The figure shows three views and two pictorial views of one solid part (mm, origin at its lowest corner). Answer the questions. Coordinates: 2 decimals unless noted, no trailing zeros. Loops run counter-clockwise (first coordinate to the right, second up) from the corner with the lowest first, then second, coordinate; pieces in that order, holes last. Notation, with made-up numbers: (23.5, -30) -> (38.5, -30) arc R12 ccw to (38.5, -26) -> close; hole circle Ø3 at (22.25, -37). An arc over 180 degrees is marked (long way). Answer as a JSON object with one key per item and string values. Group by question number.
1) Consider probe 1 along Z at (x, y) = (3, 2.3); probe 2 along X at (y, z) = (2, 32); probe 3 along Z at (x, y) = (2.45, 1.35). Determine where each line is inside the solid, lowest interval first. Write a range as [from, to].
2) Determine the mould class of the marked faces 1, 2, 3 and 4 for opening direction X: released by +X, released by -X, zero draft, split by the parting line, or undercut.
3) A flat-ended cylindrical pin translates along its axis: P1, Ø1, axis at x = 1.5, y = 2, coming from the -Z side. Find the tip coordinate at first contact, or state that the pin passes through.
4) Section A-A, the plane x = 3.8 is taken. Give the vertices of the cut face in (y, z).
5) Section B-B, the plane y = 0.45 is taken. Give the vertices of the cut face in (x, z), plus the area to 3 significant figures.
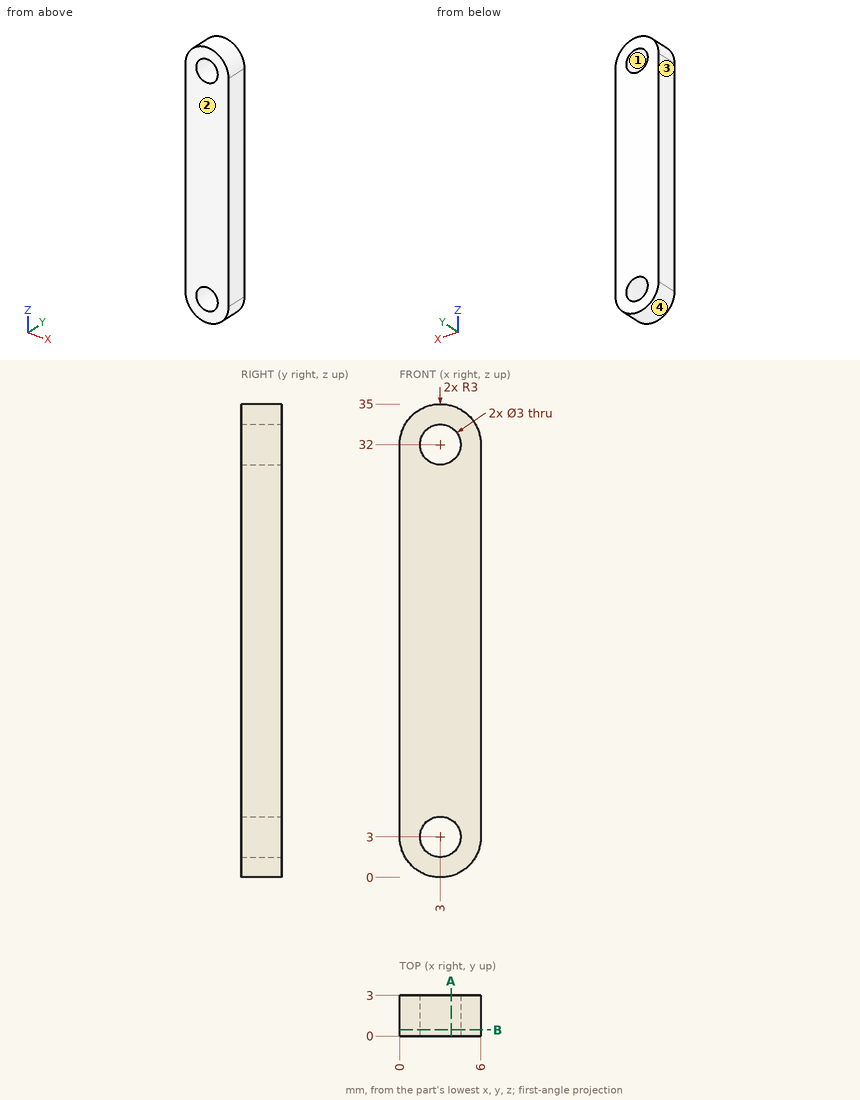
Determined:
{
 "1": {"probe 1": "[0, 1.5], [4.5, 30.5], [33.5, 35]", "probe 2": "[0, 1.5], [4.5, 6]", "probe 3": "[0.05, 1.6], [4.4, 30.6], [33.4, 34.95]"},
 "2": {"face 1": "undercut", "face 2": "zero draft", "face 3": "released by -X", "face 4": "split by the parting line"},
 "3": {"P1": "z = 0.17"},
 "4": {"outline": "(0, 0.11) -> (3, 0.11) -> (3, 1.73) -> (0, 1.73) -> close; (0, 4.27) -> (3, 4.27) -> (3, 30.73) -> (0, 30.73) -> close; (0, 33.27) -> (3, 33.27) -> (3, 34.89) -> (0, 34.89) -> close"},
 "5": {"outline": "(0, 3) arc R3 ccw to (6, 3) -> (6, 32) arc R3 ccw to (0, 32) -> close; hole circle Ø3 at (3, 3); hole circle Ø3 at (3, 32)", "area": "188 mm²"}
}
